```python
from build123d import *

# Parameters (mm, degrees)
SKETCH_1_W           = 17.78
SKETCH_1_H           = 6.35
EXTRUDE_1_DEPTH      = 5.08
SKETCH_2_W           = 16.78
SKETCH_2_H           = 5.35
CUT_EXTRUDE_1_DEPTH  = 4.08
SKETCH_3_W           = 2
SKETCH_3_H           = 4.08
CUT_EXTRUDE_2_DEPTH  = 1
EXTRUDE_2_DEPTH      = 2
EXTRUDE_2_DEPTH_BACK = 3.58
SKETCH_4_W           = 0.75
SKETCH_4_H           = 0.75


with BuildPart() as part:
    # 草图1 → 拉伸1 (new body)
    with BuildSketch(Plane(origin=(0, 0, 0), x_dir=(1, 0, 0), z_dir=(0, 1, 0))):
        Rectangle(SKETCH_1_W, SKETCH_1_H)
    extrude(amount=EXTRUDE_1_DEPTH)

    # 草图2 → 切除-拉伸1 (cut)
    with BuildSketch(Plane(origin=(0, 5.08, 0), x_dir=(-1, 0, 0), z_dir=(0, 1, 0))):
        Rectangle(SKETCH_2_W, SKETCH_2_H)
    extrude(amount=-CUT_EXTRUDE_1_DEPTH, mode=Mode.SUBTRACT)

    # 草图3 → 切除-拉伸2 (cut)
    with BuildSketch(Plane.XY.offset(3.175)):
        with Locations((0, 3.04)):
            Rectangle(SKETCH_3_W, SKETCH_3_H)
    extrude(amount=-CUT_EXTRUDE_2_DEPTH, mode=Mode.SUBTRACT)

    # 草图4 → 拉伸2 (add, two sides: drawn at the far end of the back side and taken through both)
    with BuildSketch(Plane.XZ.offset(-EXTRUDE_2_DEPTH_BACK)):
        with Locations((5.08, 0.635)):
            Rectangle(SKETCH_4_W, SKETCH_4_H)
        with Locations((0, 0.635)):
            Rectangle(SKETCH_4_W, SKETCH_4_H)
        with Locations((2.54, 0.635)):
            Rectangle(SKETCH_4_W, SKETCH_4_H)
        with Locations((7.62, 0.635)):
            Rectangle(SKETCH_4_W, SKETCH_4_H)
        with Locations((-2.54, 0.635)):
            Rectangle(SKETCH_4_W, SKETCH_4_H)
        with Locations((-7.62, 0.635)):
            Rectangle(SKETCH_4_W, SKETCH_4_H)
        with Locations((-5.08, 0.635)):
            Rectangle(SKETCH_4_W, SKETCH_4_H)
    extrude(amount=EXTRUDE_2_DEPTH + EXTRUDE_2_DEPTH_BACK)


solid = part.part
```
CAD build for the part. Positions are in the model's coordinates, mm. A direction names the side the tool comes from. Give positions to 0.01 mm unless a question says otherwise; leave off trailing zeros. Order: outer loops, then holes, each group sorted by start corner. A loop starts at its lowest first (then second) coordinate and runs counter-clockwise, first axis right, second up.
(1) Flat gauge pin, fed straight in: pin 1 (0.6 mm diameter, centred on x = -2.5, y = -1, fed in from +Z). Where does the tip first touch, or does it go through?
(2) Drill centre lines: L1, parallel to Z at x = -2.5, y = 2 (3 decimals); L2, parallel to Z at x = -3.5, y = 3.5 (3 decimals); L3, parallel to X at y = 4, z = 2. Where is each one in solid material? Low to high.
(3) Saw through at C-C, the plane y = 3.75. Give the cut face in (x, z) (3 decimals), then the cut area to 3 significant figures.
(4) Saw through at B-B, the plane x = -7. Give the cut face in (y, z) (3 decimals), then the cut area to 3 significant figures.
(5) Tool access for faces 1 (the flat face through (-5, 3, 2.675)), 2 (the flat face through (8.89, 3, 0)): list every direction of +Z, -Z, +X, -X, +Y, -Y with a clear straight run to the whole face (end or side of a thin tool).
(6) Mould opens along X. For faces 3 (the flat face through (-0.1, 0.8, 3.175)), 4 (the flat face through (-8.89, 3, 0)), 5 (the flat face through (0, 3, -2.675)) say: released by +X, released by -X, zero draft, split by the parting line, or undercut.
(7) Saw through at A-A, the plane y = -0.25. Give the cut face in (x, z) (3 decimals), then the cut area to 3 significant figures.
(8) Saw through at D-D, the plane z = -0.25. Give the cut face in (x, y), then the cut area to 3 significant figures.
Results found:
1. pin 1: stops at z = 1.01
2. L1: z = -3.175 to -2.675, 0.26 to 1.01, 2.675 to 3.175
2. L2: z = -3.175 to -2.675, 2.675 to 3.175
2. L3: x = -8.89 to -8.39, 8.39 to 8.89
3. outline: (-8.89, -3.175) - (8.89, -3.175) - (8.89, 3.175) - (1, 3.175) - (1, 2.675) - (8.39, 2.675) - (8.39, -2.675) - (-8.39, -2.675) - (-8.39, 2.675) - (-1, 2.675) - (-1, 3.175) - (-8.89, 3.175) - close
3. area: 22.1 mm2
4. outline: (0, -3.175) - (5.08, -3.175) - (5.08, -2.675) - (1, -2.675) - (1, 2.675) - (5.08, 2.675) - (5.08, 3.175) - (0, 3.175) - close
4. area: 10.4 mm2
5. face 1: +Y
5. face 2: +Z, -Z, +X, +Y, -Y
6. face 3: zero draft
6. face 4: released by -X
6. face 5: undercut
7. outline: (-7.995, 0.26) - (-7.245, 0.26) - (-7.245, 1.01) - (-7.995, 1.01) - close; (-5.455, 0.26) - (-4.705, 0.26) - (-4.705, 1.01) - (-5.455, 1.01) - close; (-2.915, 0.26) - (-2.165, 0.26) - (-2.165, 1.01) - (-2.915, 1.01) - close; (-0.375, 0.26) - (0.375, 0.26) - (0.375, 1.01) - (-0.375, 1.01) - close; (2.165, 0.26) - (2.915, 0.26) - (2.915, 1.01) - (2.165, 1.01) - close; (4.705, 0.26) - (5.455, 0.26) - (5.455, 1.01) - (4.705, 1.01) - close; (7.245, 0.26) - (7.995, 0.26) - (7.995, 1.01) - (7.245, 1.01) - close
7. area: 3.94 mm2
8. outline: (-8.89, 0) - (8.89, 0) - (8.89, 5.08) - (8.39, 5.08) - (8.39, 1) - (-8.39, 1) - (-8.39, 5.08) - (-8.89, 5.08) - close
8. area: 21.9 mm2
